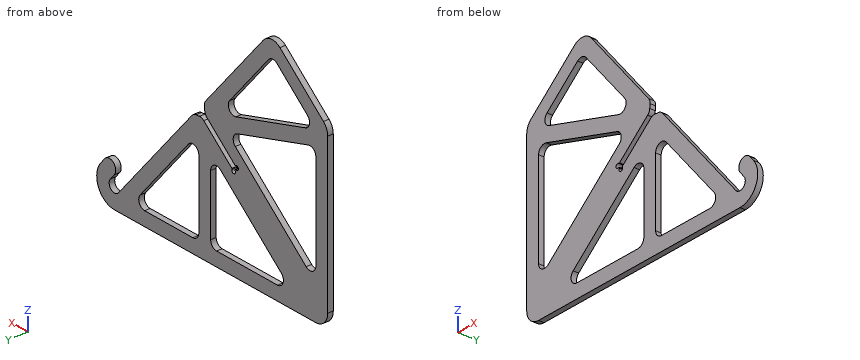
```python
from build123d import *

# Parameters (mm, degrees)
F1_DEPTH = 2
F2_SIZE  = 5
F3_R     = 5
F4_R     = 1.5
F5_DEPTH = 4.001
F6_R     = 0.5
F7_R     = 0.5
F9_DEPTH = 4.001


with BuildPart() as f1:
    # F0 (on Front) → F1 (new body, symmetric)
    with BuildSketch(Plane.XZ):
        with BuildLine():
            ThreePointArc((3.447199994, 2.8925442436), (2.8925442436, -3.447199994), (-3.447199994, -2.8925442436))
            Line((-3.447199994, -2.8925442436), (-69.9395102904, 76.349905432))
            Line((-69.9395102904, 76.349905432), (-100.5812880152, 50.6384010446))
            Line((-100.5812880152, 50.6384010446), (-103.1524384539, 53.7025788171))
            Line((-103.1524384539, 53.7025788171), (-72.5106607292, 79.4140832045))
            Line((-72.5106607292, 79.4140832045), (-125.5768458345, 142.655899949))
            ThreePointArc((-125.5768458345, 142.655899949), (-132.3657328382, 146.1899708331), (-139.6651663625, 143.8884682833))
            Line((-139.6651663625, 143.8884682833), (-176.4278760969, 113.0408921042))
            ThreePointArc((-176.4278760969, 113.0408921042), (-179.0630778704, 109.6066302904), (-180, 105.380447673))
            Line((-180, 105.380447673), (-180, -5))
            ThreePointArc((-180, -5), (-177.0710678119, -12.0710678119), (-170, -15))
            Line((-170, -15), (0, -15))
            ThreePointArc((0, -15), (13.5946168055, -6.3392739261), (11.4906666468, 9.6418141453))
            Line((11.4906666468, 9.6418141453), (8.2767285984, 13.4720363609))
            ThreePointArc((8.2767285984, 13.4720363609), (0.8803603211, 14.1191347364), (0.2332619456, 6.7227664592))
            Line((0.2332619456, 6.7227664592), (3.447199994, 2.8925442436))
        make_face()
    extrude(amount=F1_DEPTH, both=True)

    # F2
    f2_edges = [f1.edges().sort_by_distance(p)[0] for p in [
        (-72.510661, 0, 79.414083),
        (-69.93951, 0, 76.349905),
    ]]
    chamfer(f2_edges, length=F2_SIZE)

    # F3
    f3_edges = [f1.edges().sort_by_distance(p)[0] for p in [
        (-75.724599, 0, 83.244305),
        (-76.340883, 0, 76.200145),
        (-73.769733, 0, 73.135967),
        (-66.725572, 0, 72.519683),
    ]]
    fillet(f3_edges, radius=F3_R)

    # F4 (on face) → F5 (cut, through all)
    with BuildSketch(Plane.XZ.offset(2)):
        with Locations((-103.1524384539, 53.7025788171)):
            Circle(F4_R)
        with Locations((-100.5812880152, 50.6384010446)):
            Circle(F4_R)
    extrude(amount=-F5_DEPTH, mode=Mode.SUBTRACT)

    # F6
    f6_edges = [f1.edges().sort_by_distance(p)[0] for p in [
        (-102.003372, 0, 54.66676),
        (-99.432221, 0, 51.602582),
    ]]
    fillet(f6_edges, radius=F6_R)

    # F7
    f7_edges = [f1.edges().sort_by_distance(p)[0] for p in [
        (-102.188257, 0, 52.553512),
        (-101.545469, 0, 51.787468),
    ]]
    fillet(f7_edges, radius=F7_R)

    # F8 (on face) → F9 (cut, through all)
    with BuildSketch(Plane(origin=(0, 2, 0), x_dir=(-1, 0, 0), z_dir=(0, 1, 0))):
        with BuildLine():
            Line((130.0233522172, 132.3978016366), (97.2839774935, 93.3805341903))
            ThreePointArc((97.2839774935, 93.3805341903), (96.9332114879, 87.4244550998), (102.535824002, 85.3729561501))
            Line((102.535824002, 85.3729561501), (161.082054837, 102.7357001516))
            ThreePointArc((161.082054837, 102.7357001516), (164.5558221931, 106.5119215459), (162.8743685925, 111.3595623589))
            Line((162.8743685925, 111.3595623589), (137.0675124813, 133.0140858037))
            ThreePointArc((137.0675124813, 133.0140858037), (133.4177957191, 134.1648370786), (130.0233522172, 132.3978016366))
        make_face()
        with BuildLine():
            ThreePointArc((103.7888820535, 75.3140818256), (100.3151146973, 71.5378604313), (101.9965682979, 66.6902196183))
            Line((101.9965682979, 66.6902196183), (161.7860619516, 16.5208775452))
            ThreePointArc((161.7860619516, 16.5208775452), (167.1130913087, 15.8195608256), (170, 20.3510997608))
            Line((170, 20.3510997608), (170, 88.2518936709))
            ThreePointArc((170, 88.2518936709), (167.9909763068, 92.2586455639), (163.5783757071, 93.0455336626))
            Line((163.5783757071, 93.0455336626), (103.7888820535, 75.3140818256))
        make_face()
        with BuildLine():
            Line((81.1720786248, 43.1480539897), (81.1720786248, 0))
            ThreePointArc((81.1720786248, 0), (82.6365447188, -3.5355339059), (86.1720786248, -5))
            Line((86.1720786248, -5), (137.5939269804, -5))
            ThreePointArc((137.5939269804, -5), (142.2923900843, -1.7101007166), (140.8078650288, 3.8302222156))
            Line((140.8078650288, 3.8302222156), (89.3860166732, 46.9782762053))
            ThreePointArc((89.3860166732, 46.9782762053), (84.0589873161, 47.6795929249), (81.1720786248, 43.1480539897))
        make_face()
        with BuildLine():
            Line((62.3418564092, 51.7381358551), (21.6252199264, 3.2139380484))
            ThreePointArc((21.6252199264, 3.2139380484), (20.9239032068, -2.1130913087), (25.455442142, -5))
            Line((25.455442142, -5), (66.1720786248, -5))
            ThreePointArc((66.1720786248, -5), (69.7076125307, -3.5355339059), (71.1720786248, 0))
            Line((71.1720786248, 0), (71.1720786248, 48.5241978067))
            ThreePointArc((71.1720786248, 48.5241978067), (67.8821793414, 53.2226609106), (62.3418564092, 51.7381358551))
        make_face()
    extrude(amount=-F9_DEPTH, mode=Mode.SUBTRACT)


solid = f1.part
```
Check sheet for the modelled part. Datum: model origin and axes. Units: mm. Round coordinates to 2 decimals unless told otherwise and drop trailing zeros. Loops run counter-clockwise (first coordinate to the right, second up) from the corner with the lowest first, then second, coordinate; pieces in that order, holes last. Notation, with made-up numbers: (70, 45.25) - (112, 45.25) arc R21 ccw to (112, 63.25) - close; hole circle Ø9 at (7.25, 3.25). An arc over 180 degrees is marked (long way). Answer as a JSON object with one key per item and string values. Group by question number.
Q1. Sectioned sample at C-C, the plane x = -54.5. Enter the section's corners in (y, z).
Q2. Scan lines: line 1 along X through (y, z) = (-0.55, 42); line 2 along Z through (x, y) = (-122.5, 0.65); line 3 along Z through (x, y) = (-96.5, 1.65). Record each from-to range of solid material in increasing order. Write a range as [from, to].
Q3. Sectioned sample at B-B, the plane z = 122.5. Enter the section's corners in (x, y), plus the area to 3 significant figures.
Q4. Gauge pin test, flat ends, axial feed: P1, Ø2, axis at y = 1, z = 35, coming from the +X side; P2, Ø1, axis at x = -13, y = -1, coming from the +Z side; P3, Ø1, axis at y = -1, z = 14.5, coming from the +X side; P4, Ø2.5, axis at x = -100.58, z = 50.64, coming from the -Y side. Record the tip position at first contact, or that the pin passes through.
Q5. Sectioned sample at D-D, the plane y = -0.6. Count the separate pieces of the cut face and the enclosed holes in it, plus the area to 3 significant figures.
Q6. Sectioned sample at A-A, the plane x = -114.5. Enter the section's corners in (y, z), plus the area to 3 significant figures.
Solution:
{
 "1": {"outline": "(-2, -15) - (2, -15) - (2, -5) - (-2, -5) - close; (-2, 42.39) - (2, 42.39) - (2, 57.95) - (-2, 57.95) - close"},
 "2": {"line 1": "x = [-180, -170], [-131.42, -95.32], [-81.17, -71.17], [-54.17, -41.12]", "line 2": "z = [-15, -5], [19.19, 49.49], [80.86, 91.29], [123.43, 138.99]", "line 3": "z = [-15, -5], [41.01, 54.06], [59.28, 88.24], [92.09, 108]"},
 "3": {"outline": "(-165.15, -2) - (-149.6, -2) - (-149.6, 2) - (-165.15, 2) - close; (-121.72, -2) - (-108.66, -2) - (-108.66, 2) - (-121.72, 2) - close", "area": "114 mm²"},
 "4": {"P1": "stops at x = -34.4", "P2": "stops at z = 9.09", "P3": "stops at x = 7.77", "P4": "passes through"},
 "5": {"separate pieces": "1", "enclosed holes": "4", "area": "9,850 mm²"},
 "6": {"outline": "(-2, -15) - (2, -15) - (2, -5) - (-2, -5) - close; (-2, 25.91) - (2, 25.91) - (2, 56.2) - (-2, 56.2) - close; (-2, 78.49) - (2, 78.49) - (2, 88.92) - (-2, 88.92) - close; (-2, 113.9) - (2, 113.9) - (2, 129.46) - (-2, 129.46) - close", "area": "265 mm²"}
}
